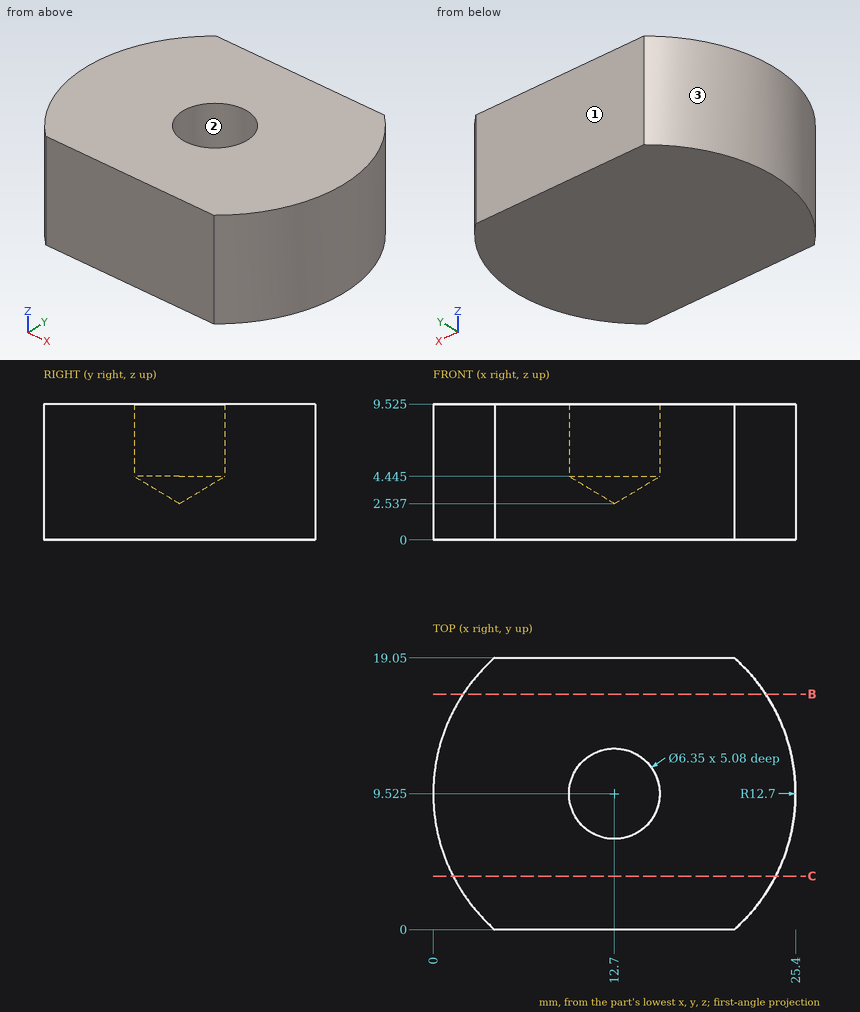
Design review of the part shown in the three views and the two pictorial views. Dimensions are in mm from the part's minimum x, y and z. Round coordinates to 2 decimals unless told otherwise and drop trailing zeros. Order: outer loops, then holes, each group sorted by start corner. A loop starts at its lowest first (then second) coordinate and runs counter-clockwise, first axis right, second up.
(1) Mouldability with a two-part tool opening along X and no side actions: class the marked faces 1, 2 and 3 as released by +X, released by -X, zero draft, split by the parting line, or undercut.
Working result:
face 1: zero draft
face 2: undercut
face 3: released by -X
(2) Take a section at B-B, the plane y = 16.5. State the section outline as (x, z) points (1 decimal), plus the area to 3 significant figures.
Working result:
outline: (2.1, 0) - (23.3, 0) - (23.3, 9.5) - (2.1, 9.5) - close
area: 202 mm2
(3) Take a section at C-C, the plane y = 3.75. State the section outline as (x, z) points (1 decimal).
Working result:
outline: (1.4, 0) - (24, 0) - (24, 9.5) - (1.4, 9.5) - close
(4) Wall thickness on L1, parallel to Y at x = 12.7, z = 7.8; L2, parallel to Y at x = 12, z = 9; L3, parallel to X at y = 2.75, z = 7: over which ranges is each line inside the solid? List them lowest first.
Working result:
L1: y = 0 to 6.35, 12.7 to 19.05
L2: y = 0 to 6.43, 12.62 to 19.05
L3: x = 1.96 to 23.44
